Autodesk Inventor part; units mm, degrees
ref_plane "YZ Plane" through (0, 0, 0) normal (1, 0, 0) x (0, 1, 0)
ref_plane "XZ Plane" through (0, 0, 0) normal (0, 1, 0) x (-1, 0, 0)
ref_plane "XY Plane" through (0, 0, 0) normal (0, 0, 1) x (1, 0, 0)
sketch "Skizze1" plane through (0, 0, 0) normal (0, 0, 1) x (1, 0, 0)
  line L0 (0, 0) -> (0, 44.5) construction
  line L1 (1.75, 0) -> (1.75, 44.5)
  line L2 (-1.75, 44.5) -> (-1.75, 0)
  arc A0 (-1.75, 0) -> (1.75, 0) centre (0, 0) ccw
  arc A1 (1.75, 44.5) -> (-1.75, 44.5) centre (0, 44.5) ccw
  point P0 (0, 22.25)
  dimension "d0" = 44.5
  dimension "d1" = 3.5
extrude "Extrusion1" add sketch "Skizze1" along normal blind 1
sketch "Skizze2" plane through (0, 0, 1) normal (0, 0, 1) x (1, 0, 0)
  arc A0 (1.75, 44.5) -> (-1.75, 44.5) centre (0, 44.5) ccw
  point P0 (0, 0)
hole "Bohrung1" at (0, 44.5, 1) at (0, 0, 1) direction (0, 0, -1) diameter 1.6 depth 1
properties part number "pleuelstange" material "Titan"
Verification items for the finished model (mm, model axes). Give positions to 0.01 mm unless a question says otherwise; leave off trailing zeros. Loops run counter-clockwise (first coordinate to the right, second up) from the corner with the lowest first, then second, coordinate; pieces in that order, holes last.
1. Material ranges on probe 1 along Y at (x, z) = (0, 0.2); probe 2 along X at (y, z) = (44.5, 0.35); probe 3 along Y at (x, z) = (-0.6, 0.2), recorded low to high.
Derived:
probe 1: y = -1.75 to -0.8, 0.8 to 43.7, 45.3 to 46.25
probe 2: x = -1.75 to -0.8, 0.8 to 1.75
probe 3: y = -1.64 to -0.53, 0.53 to 43.97, 45.03 to 46.14
2. Cross-section at B-B on z = 0.6. Record the cut outline in (x, y), and give its area (3 significant figures).
Derived:
outline: (-1.75, 0) arc R1.75 ccw to (1.75, 0) - (1.75, 44.5) arc R1.75 ccw to (-1.75, 44.5) - close; hole circle Ø1.6 at (0, 0); hole circle Ø1.6 at (0, 44.5)
area: 161 mm2
3. Go/stop test with a flat-tipped pin: P1, Ø1, axis at x = 0, y = 0, coming from the +Z side. Record where the tip stops, or that it passes through.
Derived:
P1: passes through
4. Cross-section at A-A on x = 0. Record the cut outline in (y, z).
Derived:
outline: (-1.75, 0) - (-0.8, 0) - (-0.8, 1) - (-1.75, 1) - close; (0.8, 0) - (43.7, 0) - (43.7, 1) - (0.8, 1) - close; (45.3, 0) - (46.25, 0) - (46.25, 1) - (45.3, 1) - close
5. Release check for a two-part mould opening along X. For faces 1 (the flat face through (1.75, 21.9, 0.5)), 2 (the flat face through (0, 23, 1)), 3 (the flat face through (-1.75, 22.6, 0.5)), 4 (the cylindrical face through (0.49, 0.63, 0.49)) record: +X half, -X half, draft (parallel to the pull), parting line (faces both ways), or undercut.
Derived:
face 1: +X half
face 2: draft
face 3: -X half
face 4: undercut
